Build history of the part. All positions in model axes, mm. A direction names the side the tool comes from. Give positions to 0.01 mm unless a question says otherwise; leave off trailing zeros. Order: outer loops, then holes, each group sorted by start corner. A loop starts at its lowest first (then second) coordinate and runs counter-clockwise, first axis right, second up. Notation, with made-up numbers: (60.5, 52) - (92.5, 52) arc R19 cw to (92.5, 69) - close; hole circle Ø10 at (-33.75, 58.5). An arc over 180 degrees is marked (long way). Use a Markdown table: item, result. Add a question column.
(1) Which spindle directions (+Z, -Z, +X, -X, +Y, -Y) get a long thin tool onto all of the face, cutting with end or side? Do faces 1 (the face through (33, 9, -32)), 2 (the face through (8.12, 3.7, -10.42)). Say none if no direction does.
(2) Slice it at C-C (y = 8.5). Write the cut outline in (x, z).
(3) Flat gauge pins, fed straight in: pin 1 (3 mm diameter, centred on x = 30, z = -30, fed in from +Y); pin 2 (6 mm diameter, centred on x = 10, z = -30, fed in from +Y). Where does each tip first touch, or does it go through?
(4) Slice it at B-B (x = 10). Write the cut outline in (y, z) (3 decimals), then the cut area to 3 significant figures.
(5) Slice it at A-A (y = 2). Write the cut outline in (x, z) (3 decimals).
(6) Wall check: line 1 (Z direction, x = 10, y = 5.25) (3 decimals); line 2 (X direction, y = 2.75, z = -30) (3 decimals); line 3 (X direction, y = 4.25, z = -9). Give the ranges that are in metal, low to high.
from build123d import *

# Parameters (mm, degrees)
SKETCH1_W           = 40
SKETCH1_H           = 40
SKETCH1_R           = 1.925
BOSS_EXTRUDE1_DEPTH = 10
CUT_EXTRUDE1_DEPTH  = 2.5


with BuildPart() as part:
    # Sketch1 → Boss-Extrude1 (new body)
    with BuildSketch(Plane(origin=(0, 0, 0), x_dir=(1, 0, 0), z_dir=(0, 1, 0))):
        with Locations((20, 20)):
            Rectangle(SKETCH1_W, SKETCH1_H)
        with Locations(Location((10, 30, 0), (0, 0, 270))):
            Circle(SKETCH1_R, mode=Mode.SUBTRACT)
        with Locations(Location((30, 30, 0), (0, 0, 270))):
            Circle(SKETCH1_R, mode=Mode.SUBTRACT)
        with Locations(Location((30, 10, 0), (0, 0, 270))):
            Circle(SKETCH1_R, mode=Mode.SUBTRACT)
        with Locations(Location((10, 10, 0), (0, 0, 270))):
            Circle(SKETCH1_R, mode=Mode.SUBTRACT)
    extrude(amount=BOSS_EXTRUDE1_DEPTH)

    # Sketch2 → Cut-Extrude1 (cut)
    with BuildSketch(Plane(origin=(0, 10, 0), x_dir=(1, 0, 0), z_dir=(0, 1, 0))):
        Polygon((14.156921938, 10), (12.078460969, 13.6), (7.921539031, 13.6), (5.843078062, 10), (7.921539031, 6.4), (12.078460969, 6.4), align=None)
        Polygon((25.843078062, 10), (27.921539031, 6.4), (32.078460969, 6.4), (34.156921938, 10), (32.078460969, 13.6), (27.921539031, 13.6), align=None)
        Polygon((25.843078062, 30), (27.921539031, 26.4), (32.078460969, 26.4), (34.156921938, 30), (32.078460969, 33.6), (27.921539031, 33.6), align=None)
        Polygon((14.156921938, 30), (12.078460969, 33.6), (7.921539031, 33.6), (5.843078062, 30), (7.921539031, 26.4), (12.078460969, 26.4), align=None)
    extrude(amount=-CUT_EXTRUDE1_DEPTH, mode=Mode.SUBTRACT)


solid = part.part
Solution:
| question | item | result |
|---|---|---|
| 1 | face 1 | +Y |
| 1 | face 2 | +Y, -Y |
| 2 | outline | (0, -40) - (40, -40) - (40, 0) - (0, 0) - close; hole (5.84, -30) - (7.92, -33.6) - (12.08, -33.6) - (14.16, -30) - (12.08, -26.4) - (7.92, -26.4) - close; hole (5.84, -10) - (7.92, -13.6) - (12.08, -13.6) - (14.16, -10) - (12.08, -6.4) - (7.92, -6.4) - close; hole (25.84, -30) - (27.92, -33.6) - (32.08, -33.6) - (34.16, -30) - (32.08, -26.4) - (27.92, -26.4) - close; hole (25.84, -10) - (27.92, -13.6) - (32.08, -13.6) - (34.16, -10) - (32.08, -6.4) - (27.92, -6.4) - close |
| 3 | pin 1 | through |
| 3 | pin 2 | y = 7.5 |
| 4 | outline | (0, -40) - (10, -40) - (10, -33.6) - (7.5, -33.6) - (7.5, -31.925) - (0, -31.925) - close; (0, -28.075) - (7.5, -28.075) - (7.5, -26.4) - (10, -26.4) - (10, -13.6) - (7.5, -13.6) - (7.5, -11.925) - (0, -11.925) - close; (0, -8.075) - (7.5, -8.075) - (7.5, -6.4) - (10, -6.4) - (10, 0) - (0, 0) - close |
| 4 | area | 306 mm2 |
| 5 | outline | (0, -40) - (40, -40) - (40, 0) - (0, 0) - close; hole circle Ø3.85 at (10, -30); hole circle Ø3.85 at (10, -10); hole circle Ø3.85 at (30, -30); hole circle Ø3.85 at (30, -10) |
| 6 | line 1 | -40 to -31.925, -28.075 to -11.925, -8.075 to 0 |
| 6 | line 2 | 0 to 8.075, 11.925 to 28.075, 31.925 to 40 |
| 6 | line 3 | 0 to 8.36, 11.64 to 28.36, 31.64 to 40 |
